```python
from build123d import *

# Parameters (mm, degrees)
F0_W     = 32
F0_H     = 7
F0_R     = 2.6
F0_W_2   = 2
F0_R_2   = 1.6
F1_DEPTH = 1
F2_DEPTH = 8.8
F3_DEPTH = 7.3
F4_R     = 1
F5_R     = 1


with BuildPart() as f1:
    # F0 (on Top) → F1 (new body)
    with BuildSketch(Plane.XY):
        Rectangle(F0_W, F0_H)
        Circle(F0_R, mode=Mode.SUBTRACT)
        with Locations((-17, 0)):
            Rectangle(F0_W_2, F0_H)
        with Locations((17, 0)):
            Rectangle(F0_W_2, F0_H)
        Circle(F0_R)
        Circle(F0_R_2, mode=Mode.SUBTRACT)
    extrude(amount=F1_DEPTH)

    # F0 (on Top) → F2 (join)
    with BuildSketch(Plane.XY):
        with Locations((-17, 0)):
            Rectangle(F0_W_2, F0_H)
        with Locations((17, 0)):
            Rectangle(F0_W_2, F0_H)
    extrude(amount=F2_DEPTH)

    # F0 (on Top) → F3 (join)
    with BuildSketch(Plane.XY):
        Circle(F0_R)
        Circle(F0_R_2, mode=Mode.SUBTRACT)
    extrude(amount=F3_DEPTH)

    # F4
    f4_edges = [f1.edges().sort_by_distance(p)[0] for p in [
        (-16, 0, 1),
        (16, 0, 1),
        (-18, 0, 0),
        (18, 0, 0),
        (-18, 0, 8.8),
        (18, 0, 8.8),
        (-18, -3.5, 4.4),
        (-18, 3.5, 4.4),
        (18, -3.5, 4.4),
        (18, 3.5, 4.4),
    ]]
    fillet(f4_edges, radius=F4_R)

    # F5
    f5_edges = [f1.edges().sort_by_distance(p)[0] for p in [
        (-2.6, 0, 1),
    ]]
    fillet(f5_edges, radius=F5_R)


solid = f1.part
```
Read the model definition and answer for the solid it produces. Units are mm, in the model's axes. A direction names the side the tool comes from. Give positions to 0.01 mm unless a question says otherwise; leave off trailing zeros. Order: outer loops, then holes, each group sorted by start corner. A loop starts at its lowest first (then second) coordinate and runs counter-clockwise, first axis right, second up. Notation, with made-up numbers: (85, -34) -> (129, -34) arc R19 cw to (129, -8) -> close; hole circle Ø4 at (1, 45.25). An arc over 180 degrees is marked (long way). One line per item, written item: value. Start each with the question number.
(1) Straight lines are drawn through the part: L1, parallel to Y at x = 0, z = 2.5; L2, parallel to X at y = -1, z = 4.5; L3, parallel to X at y = 2, z = 6.25. For each, find the intervals that lie inside material, in ascending order.
(2) For a pull along X with two mould halves and no side action, classify faces 1 (the flat face through (-18, 0, 4)), 2 (the flat face through (-16, 0, 5)), 3 (the flat face through (0.1, 3.5, 0.8)) as released by +X, released by -X, zero draft, split by the parting line, or undercut.
(3) The part is cut by section B-B (y = 0). Determine the outline of the cut face in (x, z), and give its area (3 significant figures).
(4) The part is cut by section A-A (z = 2.5). Determine the outline of the cut face in (x, y), and give its area (3 significant figures).
(5) A tool of negligible diameter and unlimited length cuts with its end or side. For faces 4 (the cylindrical face through (-17.699, 0.049, 0.285)), 5 (the flat face through (16, 0, 5)), from which of +Z, -Z, +X, -X, +Y, -Y can it reach the whole face along a straight path? Write none if from no direction.
(6) Flat-ended cylindrical pins translate along their axes: P1, Ø2.5, axis at x = 0, y = 0, coming from the -Z side; P2, Ø2.5, axis at x = 1, y = -0.5, coming from the +Z side; P3, Ø1, axis at x = -5, y = 2.5, coming from the +Z side; P4, Ø4, axis at x = 2.5, z = 5.5, coming from the +Y side. Find the tip coordinate at first contact, or state that the pin passes through.
(7) The part is cut by section C-C (x = -6). Determine the outline of the cut face in (y, z).
Taken from the geometry:
1. L1: -2.6 to -1.6, 1.6 to 2.6
1. L2: -18 to -16, -2.4 to -1.25, 1.25 to 2.4, 16 to 18
1. L3: -18 to -16, -1.66 to 1.66, 16 to 18
2. face 1: released by -X
2. face 2: undercut
2. face 3: zero draft
3. outline: (-18, 1) arc R1 ccw to (-17, 0) -> (-1.6, 0) -> (-1.6, 7.3) -> (-2.6, 7.3) -> (-2.6, 2) arc R1 cw to (-3.6, 1) -> (-15, 1) arc R1 cw to (-16, 2) -> (-16, 8.8) -> (-17, 8.8) arc R1 ccw to (-18, 7.8) -> close; (1.6, 0) -> (17, 0) arc R1 ccw to (18, 1) -> (18, 7.8) arc R1 ccw to (17, 8.8) -> (16, 8.8) -> (16, 2) arc R1 cw to (15, 1) -> (3.6, 1) arc R1 cw to (2.6, 2) -> (2.6, 7.3) -> (1.6, 7.3) -> close
3. area: 76.6 mm^2
4. outline: (-18, -2.5) arc R1 ccw to (-17, -3.5) -> (-16, -3.5) -> (-16, 3.5) -> (-17, 3.5) arc R1 ccw to (-18, 2.5) -> close; circle Ø5.2 at (0, 0); (16, -3.5) -> (17, -3.5) arc R1 ccw to (18, -2.5) -> (18, 2.5) arc R1 ccw to (17, 3.5) -> (16, 3.5) -> close; hole circle Ø3.2 at (0, 0)
4. area: 40.3 mm^2
5. face 4: -Z, -X, +Y, -Y
5. face 5: +Z, +Y, -Y
6. P1: through
6. P2: z = 7.3
6. P3: z = 1
6. P4: y = 2.55
7. outline: (-3.5, 0) -> (3.5, 0) -> (3.5, 1) -> (-3.5, 1) -> close
